from build123d import *

# Parameters (mm, degrees)
F0_R     = 29.21
F0_R_2   = 25.4
F1_DEPTH = 50.8
F0_R_3   = 38.1
F2_DEPTH = 12.7
F3_R     = 3.175
F4_DEPTH = 12.7
F5_R     = 38.1
F5_R_2   = 25.4
F6_DEPTH = 2.54


with BuildPart() as f1:
    # F0 (on Front) → F1 (new body)
    with BuildSketch(Plane.XZ):
        Circle(F0_R)
        Circle(F0_R_2, mode=Mode.SUBTRACT)
    extrude(amount=F1_DEPTH)

    # F0 (on Front) → F2 (join)
    with BuildSketch(Plane.XZ):
        Circle(F0_R_3)
        Circle(F0_R, mode=Mode.SUBTRACT)
    extrude(amount=F2_DEPTH)

    # F3 (on face) → F4 (cut)
    with BuildSketch(Plane.XZ):
        with Locations((-31.75, 0)):
            Circle(F3_R)
        with Locations((-15.875, -27.496307)):
            Circle(F3_R)
        with Locations((15.875, -27.496307)):
            Circle(F3_R)
        with Locations((31.75, 0)):
            Circle(F3_R)
        with Locations((15.875, 27.496307)):
            Circle(F3_R)
        with Locations((-15.875, 27.496307)):
            Circle(F3_R)
    extrude(amount=F4_DEPTH, mode=Mode.SUBTRACT)

    # F5 (on face) → F6 (join)
    with BuildSketch(Plane.XZ.offset(50.8)):
        Circle(F5_R)
        Circle(F5_R_2, mode=Mode.SUBTRACT)
    extrude(amount=-F6_DEPTH)


solid = f1.part
Design review of the part built by this model. Coordinates are the model's own, in mm. A direction names the side the tool comes from. Round coordinates to 2 decimals unless told otherwise and drop trailing zeros. Loops run counter-clockwise (first coordinate to the right, second up) from the corner with the lowest first, then second, coordinate; pieces in that order, holes last. Notation, with made-up numbers: (39.25, 87) - (97.25, 87) arc R36 cw to (97.25, 122) - close; hole circle Ø6 at (27.5, 68). An arc over 180 degrees is marked (long way). One line per question, with ' | ' between items.
1. Clearance check with flat-ended pins moving along their axes: P1, Ø1, axis at x = -7.5, z = -29.5, coming from the +Y side; P2, Ø5, axis at x = 27, y = -39, coming from the +Z side; P3, Ø0.9, axis at x = 15, z = 25, coming from the +Y side; P4, Ø3, axis at x = -12.5, y = -32.5, coming from the -Z side. State where each tip first meets the part, or that it passes through.
Results are:
P1: stops at y = 0 | P2: stops at z = 15.91 | P3: stops at y = -12.7 | P4: stops at z = -27.06
2. We need section A-A, the plane x = 0. State the section outline as (y, z) points, and give its area (3 significant figures).
Results are:
outline: (-50.8, -38.1) - (-48.26, -38.1) - (-48.26, -29.21) - (-12.7, -29.21) - (-12.7, -38.1) - (0, -38.1) - (0, -25.4) - (-50.8, -25.4) - close; (-50.8, 25.4) - (0, 25.4) - (0, 38.1) - (-12.7, 38.1) - (-12.7, 29.21) - (-48.26, 29.21) - (-48.26, 38.1) - (-50.8, 38.1) - close | area: 658 mm²
3. We need section D-D, the plane y = -45. State the section outline as (x, z) points, and give its area (3 significant figures).
Results are:
outline: circle Ø58.42 at (0, 0); hole circle Ø50.8 at (0, 0) | area: 654 mm²
4. For faces 4 (the face through (-5.506, -25.044, -24.796)), 5 (the face through (18.903, -6.261, 28.45)), 6 (the face through (-9, -48.26, -28)), list the 3-axis set-ups (+Z, -Z, +X, -X, +Y, -Y) from which the entire face can be reached by the end or side of a thin tool; tool diameter is ignored.
Results are:
face 4: +Y, -Y | face 5: +Y | face 6: none
5. We need section B-B, the plane z = 0. State the section outline as (x, y) points (3 decimals).
Results are:
outline: (-38.1, -50.8) - (-25.4, -50.8) - (-25.4, 0) - (-28.575, 0) - (-28.575, -12.7) - (-29.21, -12.7) - (-29.21, -48.26) - (-38.1, -48.26) - close; (-38.1, -12.7) - (-34.925, -12.7) - (-34.925, 0) - (-38.1, 0) - close; (25.4, -50.8) - (38.1, -50.8) - (38.1, -48.26) - (29.21, -48.26) - (29.21, -12.7) - (28.575, -12.7) - (28.575, 0) - (25.4, 0) - close; (34.925, -12.7) - (38.1, -12.7) - (38.1, 0) - (34.925, 0) - close
6. Draft analysis for pull direction Z (two halves, no side actions). For faces 1 (the face through (-9, -12.7, -28)), 2 (the face through (15.46, -6.26, -24.35)), 3 (the face through (-30.235, -6.261, -23.183)), state which applies: released by +Z, released by -Z, zero draft, split by the parting line, or undercut.
Results are:
face 1: zero draft | face 2: undercut | face 3: split by the parting line
7. We need section C-C, the plane z = 33. State the section outline as (x, y) points.
Results are:
outline: (-19.04, -50.8) - (19.04, -50.8) - (19.04, -48.26) - (-19.04, -48.26) - close; (-19.04, -12.7) - (19.04, -12.7) - (19.04, 0) - (-19.04, 0) - close
8. For L1, parallel to Y at x = 22.5, z = 30; L2, parallel to Z at x = 16, y = -4.5; L3, parallel to Z at x = 0, y = -33, list the stretches that pass through material, from the lowest coordinate up. Write a range as [from, to].
Results are:
L1: y = [-50.8, -48.26], [-12.7, 0] | L2: z = [-34.58, -30.67], [-24.32, -19.73], [19.73, 24.32], [30.67, 34.58] | L3: z = [-29.21, -25.4], [25.4, 29.21]
